Input: part model. Units: mm. Frame: model coordinates. A direction names the side the tool comes from. Give positions to 0.01 mm unless a question says otherwise; leave off trailing zeros. Write each loop counter-clockwise with the first axis right and the second up, starting at its lowest first coordinate (ties: lowest second). Pieces come first, ordered by that corner, then holes. Notation, with made-up numbers: (84.25, -4) -> (119.25, -4) arc R8 cw to (119.25, 2) -> close; hole circle Ø1 at (19.25, 86). An arc over 180 degrees is marked (long way). Answer as a JSON object with one key per item and string values. Group by question number.
from build123d import *

# Parameters (mm, degrees)
EXTRUDE_THIN1_DEPTH            = 510
EXTRUDE_THIN1_DEPTH_BACK       = 290
SKETCH1_W                      = 76.2
SKETCH1_H                      = 38.1
SKETCH1_W_2                    = 69.85
SKETCH1_H_2                    = 31.75
F_12_0_12_DIAMETER_HOLE1_D     = 12
F_12_0_12_DIAMETER_HOLE1_DEPTH = 3.175
CUT_EXTRUDE1_REACH             = 514.838
SKETCH6_R                      = 17.5
CUT_EXTRUDE2_REACH             = 514.838
SKETCH7_R                      = 17.5


with BuildPart() as part:
    # Sketch1 → Extrude-Thin1 (new, two sides: drawn at the far end of the back side and taken through both)
    with BuildSketch(Plane(origin=(0, 0, 0), x_dir=(1, 0, 0), z_dir=(0, 1, 0)).offset(-EXTRUDE_THIN1_DEPTH_BACK)):
        Rectangle(SKETCH1_W, SKETCH1_H)
        Rectangle(SKETCH1_W_2, SKETCH1_H_2, mode=Mode.SUBTRACT)
    extrude(amount=EXTRUDE_THIN1_DEPTH + EXTRUDE_THIN1_DEPTH_BACK)

    # Ø12.0 (12) Diameter Hole1
    with Locations(Plane(origin=(0, 0, -19.05), x_dir=(-1, 0, 0), z_dir=(0, 0, -1))):
        with Locations((-20, -25), (20, -275), (-20, -275), (20, -25)):
            Hole(F_12_0_12_DIAMETER_HOLE1_D / 2, depth=F_12_0_12_DIAMETER_HOLE1_DEPTH)

    # Sketch6 → Cut-Extrude1 (cut, up to next)
    with BuildSketch(Plane.XY.offset(19.05), mode=Mode.PRIVATE) as cut_extrude1_sk1:
        with Locations((0, 475)):
            Circle(SKETCH6_R)
    cut_extrude1_tool1 = extrude(cut_extrude1_sk1.sketch, amount=-CUT_EXTRUDE1_REACH, mode=Mode.PRIVATE) & part.part
    add(cut_extrude1_tool1.solids().sort_by_distance((0, 475, 19.05))[0], mode=Mode.SUBTRACT)

    # Sketch7 → Cut-Extrude2 (cut, up to next)
    with BuildSketch(Plane(origin=(0, 0, -19.05), x_dir=(-1, 0, 0), z_dir=(0, 0, -1)), mode=Mode.PRIVATE) as cut_extrude2_sk1:
        with Locations((0, -75)):
            Circle(SKETCH7_R)
    cut_extrude2_tool1 = extrude(cut_extrude2_sk1.sketch, amount=-CUT_EXTRUDE2_REACH, mode=Mode.PRIVATE) & part.part
    add(cut_extrude2_tool1.solids().sort_by_distance((0, -75, -19.05))[0], mode=Mode.SUBTRACT)


solid = part.part
1. Section A-A (z = 7). Return the cut outline in (x, y) (3 decimals).
2. Line query: line 1 (X direction, y = -275, z = -17.6); line 2 (Y direction, x = 20, z = -16.5); line 3 (Z direction, x = -27, y = 75.5) (3 decimals). Output: solid intervals per line, ascending.
3. Reachability of faces 1 (the face through (3.794, -92.084, -17.485)), 2 (the face through (-1, 104, -19.05)), 3 (the face through (0, 104, 15.875)) from +Z, -Z, +X, -X, +Y, -Y: full face, straight path, thin tool, end or side. Return the list, or none.
4. Section B-B (x = 0). Return the cut outline in (y, z) (3 decimals), plus the area to 3 significant figures.
5. Mould query, pull axis Y, two halves, no side actions, for faces 4 (the face through (-3, -290, 17)), 5 (the face through (-1, 104, 19.05)), 6 (the face through (-2.28, 492.35, 17.48)). Classes: pulls with the +Y half, pulls with the -Y half, needs draft (parallel to the pull), parting line crosses it, or undercut.
6. Section C-C (y = -75). Return the cut outline in (x, z) (3 decimals).
Working result:
{
 "1": {"outline": "(-38.1, -290) -> (-34.925, -290) -> (-34.925, 510) -> (-38.1, 510) -> close; (34.925, -290) -> (38.1, -290) -> (38.1, 510) -> (34.925, 510) -> close"},
 "2": {"line 1": "x = -38.1 to -26, -14 to 14, 26 to 38.1", "line 2": "y = -290 to -281, -269 to -31, -19 to 510", "line 3": "z = -19.05 to -15.875, 15.875 to 19.05"},
 "3": {"face 1": "-Z", "face 2": "-Z, +X, -X, +Y, -Y", "face 3": "+Y, -Y"},
 "4": {"outline": "(-290, -19.05) -> (-92.5, -19.05) -> (-92.5, -15.875) -> (-290, -15.875) -> close; (-290, 15.875) -> (457.5, 15.875) -> (457.5, 19.05) -> (-290, 19.05) -> close; (-57.5, -19.05) -> (510, -19.05) -> (510, -15.875) -> (-57.5, -15.875) -> close; (492.5, 15.875) -> (510, 15.875) -> (510, 19.05) -> (492.5, 19.05) -> close", "area": "4,860 mm^2"},
 "5": {"face 4": "pulls with the -Y half", "face 5": "needs draft", "face 6": "undercut"},
 "6": {"outline": "(-38.1, -19.05) -> (-17.5, -19.05) -> (-17.5, -15.875) -> (-34.925, -15.875) -> (-34.925, 15.875) -> (34.925, 15.875) -> (34.925, -15.875) -> (17.5, -15.875) -> (17.5, -19.05) -> (38.1, -19.05) -> (38.1, 19.05) -> (-38.1, 19.05) -> close"}
}
